```python
from build123d import *

# Parameters (mm, degrees)
SKETCH1_W           = 177.8
SKETCH1_H           = 19.05
BOSS_EXTRUDE1_DEPTH = 6.35
SKETCH2_W           = 12.7
SKETCH2_H           = 6.35
BOSS_EXTRUDE2_DEPTH = 6.35
SKETCH3_W           = 12.7
SKETCH3_H           = 6.35
BOSS_EXTRUDE3_DEPTH = 6.35


with BuildPart() as part:
    # Sketch1 → Boss-Extrude1 (new body)
    with BuildSketch(Plane.XY):
        with Locations((88.9, 9.525)):
            Rectangle(SKETCH1_W, SKETCH1_H)
    extrude(amount=BOSS_EXTRUDE1_DEPTH)

    # Sketch2 → Boss-Extrude2 (add)
    with BuildSketch(Plane(origin=(0, 19.05, 0), x_dir=(1, 0, 0), z_dir=(0, 1, 0))):
        with Locations((31.75, -3.175)):
            Rectangle(SKETCH2_W, SKETCH2_H)
        with Locations((146.05, -3.175)):
            Rectangle(SKETCH2_W, SKETCH2_H)
    extrude(amount=BOSS_EXTRUDE2_DEPTH)

    # Sketch3 → Boss-Extrude3 (add)
    with BuildSketch(Plane.XZ):
        with Locations((31.75, 3.175)):
            Rectangle(SKETCH3_W, SKETCH3_H)
        with Locations((146.05, 3.175)):
            Rectangle(SKETCH3_W, SKETCH3_H)
    extrude(amount=BOSS_EXTRUDE3_DEPTH)


solid = part.part
```
Here's how the part is built. I have some questions about the finished solid (model axes, mm). A direction names the side the tool comes from. Round coordinates to 2 decimals unless told otherwise and drop trailing zeros. Order: outer loops, then holes, each group sorted by start corner. A loop starts at its lowest first (then second) coordinate and runs counter-clockwise, first axis right, second up. Notation, with made-up numbers: M 41,-21.75 L 63,-21.75 A11 ccw 63,-14.75 Z; hole C 84.5,-6.5 d8. An arc over 180 degrees is marked long. Use CSV: the item, a comma, the result in double quotes.
1) I want a section at C-C (x = 17.5). List the corners of the cut face in (y, z) for me.
Taken from the geometry:
outline,"M 0,0 L 19.05,0 L 19.05,6.35 L 0,6.35 Z"
2) I'm going to push flat-ended pins straight in: P1, Ø3, axis at y = -3.5, z = 1.5, coming from the +X side; P2, Ø3, axis at x = 11.5, z = 3.5, coming from the -Y side; P3, Ø12, axis at x = 20, y = -3, coming from the -Z side; P4, Ø3, axis at x = 14, z = 4, coming from the +Y side. Where does each tip first touch, or does it pass through?
Taken from the geometry:
P1,"x = 152.4"
P2,"y = 0"
P3,"z = 0"
P4,"y = 19.05"
3) If we mould it in two halves opening along X, with no side actions, what happens to faces 1 (the flat face through (139.7, 22, 3)), 2 (the flat face through (25.4, -3, 3)), 3 (the flat face through (32, 25.4, 3))? For each: pulls with the +X half, pulls with the -X half, needs draft (parallel to the pull), parting line crosses it, or undercut.
Taken from the geometry:
face 1,"undercut"
face 2,"pulls with the -X half"
face 3,"needs draft"
4) On a 3-axis mill with a long thin cutter (end or side, diameter ignored), from which of +Z, -Z, +X, -X, +Y, -Y can I reach the whole of each face in a straight line? I mean faces 4 (the flat face through (38.1, -3, 3)), 5 (the flat face through (13, 19.05, 3)), 6 (the flat face through (38.1, 22, 3)), 7 (the flat face through (165, 19.05, 3)). Say none if no direction works.
Taken from the geometry:
face 4,"+Z, -Z, -Y"
face 5,"+Z, -Z, -X, +Y"
face 6,"+Z, -Z, +Y"
face 7,"+Z, -Z, +X, +Y"
5) I want a section at B-B (z = 1.25). List the corners of the cut face in (x, y) for me, then the cut area to 3 significant figures.
Taken from the geometry:
outline,"M 0,0 L 25.4,0 L 25.4,-6.35 L 38.1,-6.35 L 38.1,0 L 139.7,0 L 139.7,-6.35 L 152.4,-6.35 L 152.4,0 L 177.8,0 L 177.8,19.05 L 152.4,19.05 L 152.4,25.4 L 139.7,25.4 L 139.7,19.05 L 38.1,19.05 L 38.1,25.4 L 25.4,25.4 L 25.4,19.05 L 0,19.05 Z"
area,"3,710 mm^2"
6) I need wall thicknesses on line 1 along X through (y, z) = (23, 4.5); line 2 along Y through (x, z) = (45, 3.5). Which ranges of each line are inside material? Lowest first, please. Write a range as [from, to].
Taken from the geometry:
line 1,"[25.4, 38.1], [139.7, 152.4]"
line 2,"[0, 19.05]"
7) I want a section at A-A (y = 20.5). List the corners of the cut face in (x, z) for me, then the cut area to 3 significant figures.
Taken from the geometry:
outline,"M 25.4,0 L 38.1,0 L 38.1,6.35 L 25.4,6.35 Z; M 139.7,0 L 152.4,0 L 152.4,6.35 L 139.7,6.35 Z"
area,"161 mm^2"
